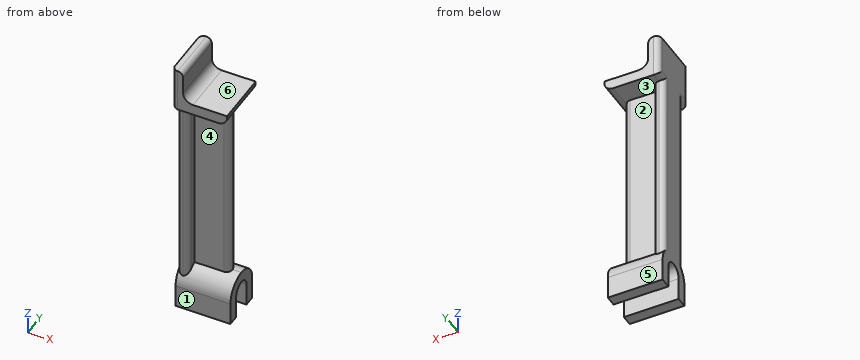
from build123d import *

# Parameters (mm, degrees)
F1_DEPTH = 12.5
F3_DEPTH = 25
F4_W     = 16
F4_H     = 5
F5_DEPTH = 89.876524617
F6_R     = 3.99999
F7_R     = 2.4999


# Not quite as in the source:
# - a fillet or chamfer is up to 0.001 mm smaller than in the source, because OpenCascade refuses the exact size


with BuildPart() as f1:
    # F0 (on Front) → F1 (new body, symmetric)
    with BuildSketch(Plane.XZ):
        with BuildLine():
            ThreePointArc((0, 100), (-3.1819805153, 101.3180194847), (-4.5, 104.5))
            Line((-4.5, 104.5), (-4.5, 115))
            Line((-4.5, 115), (-9.5, 115))
            Line((-9.5, 115), (-9.5, 95))
            Line((-9.5, 95), (15.5, 95))
            Line((15.5, 95), (15.5, 100))
            Line((15.5, 100), (0, 100))
        make_face()
    extrude(amount=F1_DEPTH, both=True)



with BuildPart() as f3:
    # F2 (on face) → F3 (new body)
    with BuildSketch(Plane(origin=(-9.5, 0, 0), x_dir=(0, -1, 0), z_dir=(-1, 0, 0))):
        with BuildLine():
            ThreePointArc((-4.5, 0), (0, 4.5), (4.5, 0))
            Line((4.5, 0), (4.5, -10.5))
            Line((4.5, -10.5), (9.5, -10.5))
            Line((9.5, -10.5), (9.5, 0))
            ThreePointArc((9.5, 0), (6.7175144213, 6.7175144213), (0, 9.5))
            ThreePointArc((0, 9.5), (-6.7175144213, 6.7175144213), (-9.5, 0))
            Line((-9.5, 0), (-9.5, -10.5))
            Line((-9.5, -10.5), (-4.5, -10.5))
            Line((-4.5, -10.5), (-4.5, 0))
        make_face()
    extrude(amount=-F3_DEPTH)


with BuildPart() as f1_1:
    add(f1.part)

    add(f3.part)  # F5 merges F3
    # F4 (on face) → F5 (join, through all)
    with BuildSketch(Plane(origin=(0, 0, 95), x_dir=(1, 0, 0), z_dir=(0, 0, -1))):
        Polygon((-4.5, 8), (-9.5, 8), (-9.5, -8), (-4.5, -8), (-4.5, -2.5), (-4.5, 2.5), align=None)
        with Locations((3.5, 0)):
            Rectangle(F4_W, F4_H)
    extrude(amount=F5_DEPTH)

    # F6 (radius 4 in the source; OpenCascade refuses exactly that, so slightly less here)
    f6_edges = [f1_1.edges().sort_by_distance(p)[0] for p in [
        (15.5, 0, 95),
    ]]
    fillet(f6_edges, radius=F6_R)

    # F7 (radius 2.5 in the source; OpenCascade refuses exactly that, so slightly less here)
    f7_edges = [f1_1.edges().sort_by_distance(p)[0] for p in [
        (11.5, -2.5, 52.082576),
        (11.5, 2.5, 52.082576),
        (-4.5, -8, 50.061738),
        (-4.5, 8, 50.061738),
        (-9.5, 8, 50.061738),
        (-9.5, -8, 50.061738),
        (-9.5, -10.25, 95),
        (-9.5, 10.25, 95),
        (-9.5, -12.5, 105),
        (-9.5, 12.5, 105),
        (-4.5, 0, 115),
    ]]
    fillet(f7_edges, radius=F7_R)


solid = f1_1.part
Read the model definition and answer for the solid it produces. Units are mm, in the model's axes. Face numbers are marked on the shaded views. A direction names the side the tool comes from. Round coordinates to 2 decimals unless told otherwise and drop trailing zeros. Order: outer loops, then holes, each group sorted by start corner. A loop starts at its lowest first (then second) coordinate and runs counter-clockwise, first axis right, second up.
1) The part is cut by section C-C on y = 1.25. Write down the section's boundary in (x, z), plus the area to 3 significant figures.
2) The mould has two halves that part along Z. Classify the marked faces 4, 5 and 6: released by +Z, released by -Z, zero draft, split by the parting line, or undercut.
3) For the marked faces 1, 2 and 3, determine the directions among +Z, -Z, +X, -X, +Y, -Y from which every point of the face is accessible in a straight line to the end or side of a thin tool.
4) Straight lines are drawn through the part: L1, parallel to Y at x = 4.5, z = 42; L2, parallel to X at y = 5, z = 46; L3, parallel to Z at x = 13.75, y = 0.75. For each, find the intervals that lie inside material, in ascending order.
5) Flat-ended cylindrical pins translate along their axes: pin 1 (5 mm diameter, centred on x = -0.5, y = -1, fed in from +Z); pin 2 (12.5 mm diameter, centred on x = 6.5, y = -3, fed in from +Z); pin 3 (5 mm diameter, centred on x = 6, z = -5.5, fed in from -Y). Find the tip coordinate at first contact, or state that the pin passes through.
6) The part is cut by section B-B on x = -3. Write down the section's boundary in (y, z), plus the area to 3 significant figures.
Resolved:
1. outline: (-9.5, 4.32) - (15.5, 4.32) - (15.5, 9.42) - (11.17, 9.42) - (11.17, 95) - (11.5, 95) arc R4 ccw to (15.5, 99) - (15.5, 100) - (0, 100) arc R4.5 cw to (-4.5, 104.5) - (-4.5, 112.5) arc R2.5 ccw to (-7, 115) - (-9.5, 115) - close
1. area: 2,100 mm2
2. face 4: undercut
2. face 5: zero draft
2. face 6: released by +Z
3. face 1: -Z, +X, -X, -Y
3. face 2: +X, +Y
3. face 3: +X, +Y
4. L1: y = -2.5 to 2.5
4. L2: x = -9.5 to -4.5
4. L3: z = 4.44 to 9.47, 95.69 to 100
5. pin 1: stops at z = 101.15
5. pin 2: stops at z = 100
5. pin 3: stops at y = -9.5
6. outline: (-12.5, 95) - (-2.5, 95) - (-2.5, 9.17) arc R9.5 ccw to (-9.5, 0) - (-9.5, -10.5) - (-4.5, -10.5) - (-4.5, 0) arc R4.5 cw to (4.5, 0) - (4.5, -10.5) - (9.5, -10.5) - (9.5, 0) arc R9.5 ccw to (2.5, 9.17) - (2.5, 95) - (12.5, 95) - (12.5, 101.15) - (-12.5, 101.15) - close
6. area: 797 mm2
